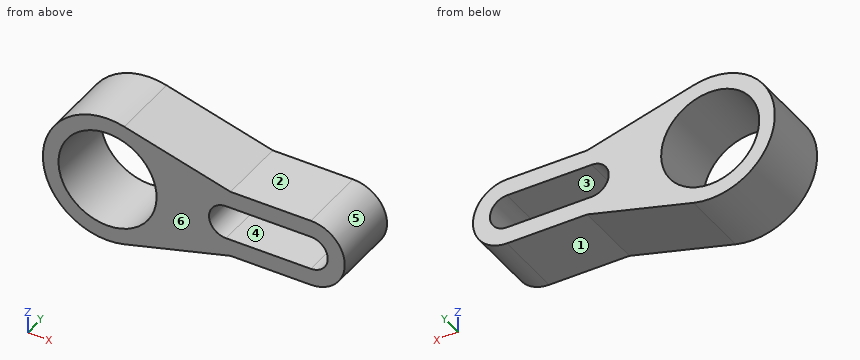
from build123d import *

# Parameters (mm, degrees)
SKETCH1_R           = 9.145
BOSS_EXTRUDE3_DEPTH = 13


with BuildPart() as part:
    # Sketch1 → Boss-Extrude3 (new body)
    with BuildSketch(Plane(origin=(0, 0, 0), x_dir=(1, 0, 0), z_dir=(0, 1, 0))):
        with BuildLine():
            Line((22.935251834, 6.35), (3.119976244, 11.654611672))
            ThreePointArc((3.119976244, 11.654611672), (-12.065, 0), (3.119976244, -11.654611672))
            Line((3.119976244, -11.654611672), (22.935251834, -6.35))
            Line((22.935251834, -6.35), (37.9, -6.35))
            ThreePointArc((37.9, -6.35), (44.25, 0), (37.9, 6.35))
            Line((37.9, 6.35), (22.935251834, 6.35))
        make_face()
        with Locations(Location((0, 0, 0), (0, 0, 90))):
            Circle(SKETCH1_R, mode=Mode.SUBTRACT)
        with BuildLine():
            Line((37.9, -3.175), (22.1, -3.175))
            ThreePointArc((22.1, -3.175), (18.925, 0), (22.1, 3.175))
            Line((22.1, 3.175), (37.9, 3.175))
            ThreePointArc((37.9, 3.175), (41.075, 0), (37.9, -3.175))
        make_face(mode=Mode.SUBTRACT)
    extrude(amount=BOSS_EXTRUDE3_DEPTH)


solid = part.part
Geometry check sheet. Reference: the model listing, model coordinates, mm. Face numbers are marked on the shaded views. A direction names the side the tool comes from. Round coordinates to 2 decimals unless told otherwise and drop trailing zeros. Order: outer loops, then holes, each group sorted by start corner. A loop starts at its lowest first (then second) coordinate and runs counter-clockwise, first axis right, second up. Notation, with made-up numbers: (-38.5, 89.25) -> (-28.5, 89.25) arc R12 cw to (-28.5, 111.25) -> close; hole circle Ø5 at (30, 48.25). An arc over 180 degrees is marked (long way). Use one line per item in the form item = value.
1. Go/stop test with flat-tipped pins: pin 1 (6 mm diameter, centred on x = 6.5, y = 10.5, fed in from -Z); pin 2 (6.5 mm diameter, centred on x = 32, y = 9, fed in from -Z); pin 3 (2 mm diameter, centred on x = 11, y = 10, fed in from -Z). Record where each tip stops, or that it passes through.
Working result:
pin_1 = -11.55
pin_2 = -6.35
pin_3 = -9.81
2. Cross-section at B-B, the plane y = 8. Enter the section's corners in (x, z) (3 decimals).
Working result:
outline = (3.12, -11.655) -> (22.935, -6.35) -> (37.9, -6.35) arc R6.35 ccw to (37.9, 6.35) -> (22.935, 6.35) -> (3.12, 11.655) arc R12.065 ccw (long way) to start; hole circle Ø18.29 at (0, 0); hole (22.1, -3.175) -> (37.9, -3.175) arc R3.175 ccw to (37.9, 3.175) -> (22.1, 3.175) arc R3.175 ccw to start
3. Cross-section at D-D, the plane z = 5.75. Enter the section's corners in (x, y), plus the area to 3 significant figures.
Working result:
outline = (-10.61, 0) -> (-7.11, 0) -> (-7.11, 13) -> (-10.61, 13) -> close; (7.11, 0) -> (40.59, 0) -> (40.59, 13) -> (7.11, 13) -> close
area = 481 mm^2
4. Mould release check, pull along X, two halves, no side actions. Record for the marked faces 4, 5 and 6: pulls with the +X half, pulls with the -X half, needs draft (parallel to the pull), parting line crosses it, or undercut.
Working result:
face_4 = undercut
face_5 = pulls with the +X half
face_6 = needs draft
5. Set-up check for the marked faces 1, 2 and 3: record each of +Z, -Z, +X, -X, +Y, -Y from which the full face is reachable in a straight line by a thin tool's end or side.
Working result:
face_1 = -Z, +X, +Y, -Y
face_2 = +Z, +X, +Y, -Y
face_3 = +Y, -Y
6. Cross-section at C-C, the plane z = 0. Enter the section's corners in (x, y) (3 decimals), plus the area to 3 significant figures.
Working result:
outline = (-12.065, 0) -> (-9.145, 0) -> (-9.145, 13) -> (-12.065, 13) -> close; (9.145, 0) -> (18.925, 0) -> (18.925, 13) -> (9.145, 13) -> close; (41.075, 0) -> (44.25, 0) -> (44.25, 13) -> (41.075, 13) -> close
area = 206 mm^2
7. Cross-section at A-A, the plane x = 26. Enter the section's corners in (y, z) (3 decimals).
Working result:
outline = (0, -6.35) -> (13, -6.35) -> (13, -3.175) -> (0, -3.175) -> close; (0, 3.175) -> (13, 3.175) -> (13, 6.35) -> (0, 6.35) -> close
8. Scan lines: line 1 along X through (y, z) = (6, 0) (3 decimals); line 2 along Z through (x, y) = (31.5, 2) (3 decimals); line 3 along X through (y, z) = (1.5, -1.75). Record each from-to range of solid material in increasing order. Write a range as from..to.
Working result:
line_1 = -12.065..-9.145, 9.145..18.925, 41.075..44.25
line_2 = -6.35..-3.175, 3.175..6.35
line_3 = -11.94..-8.98, 8.98..19.45, 40.55..44
